```python
from build123d import *

# Parameters (mm, degrees)
SKETCH1_W           = 150
SKETCH1_H           = 150
SKETCH1_W_2         = 140
SKETCH1_H_2         = 140
BOSS_EXTRUDE1_DEPTH = 80
BOSS_EXTRUDE2_DEPTH = 2
CIRPATTERN1_COUNT   = 4
CUT_EXTRUDE1_DEPTH  = 10


with BuildPart() as part:
    # Sketch1 → Boss-Extrude1 (new body)
    with BuildSketch(Plane(origin=(0, 91.979453816, 0), x_dir=(1, 0, 0), z_dir=(0, 1, 0))):
        with Locations((62.661143414, -111.558685069)):
            Rectangle(SKETCH1_W, SKETCH1_H)
        with Locations((62.661143414, -111.558685069)):
            Rectangle(SKETCH1_W_2, SKETCH1_H_2, mode=Mode.SUBTRACT)
    extrude(amount=BOSS_EXTRUDE1_DEPTH)

    # Sketch5 → Boss-Extrude2 (add)
    with BuildSketch(Plane.XZ.offset(-91.979453816)):
        with BuildLine():
            Line((-8.863856586, 184.058685069), (-8.863856586, 39.058685069))
            ThreePointArc((-8.863856586, 39.058685069), (-9.838856586, 38.083685069), (-10.813856586, 39.058685069))
            Line((-10.813856586, 39.058685069), (-10.813856586, 184.058685069))
            ThreePointArc((-10.813856586, 184.058685069), (-9.838856586, 185.033685069), (-8.863856586, 184.058685069))
        make_face()
    boss_extrude2 = extrude(amount=BOSS_EXTRUDE2_DEPTH)

    # CirPattern1: Boss-Extrude2 ×4 about axis
    cirpattern1_axis = Axis((62.661143414, 0, 111.558685069), (0, 1, 0))
    for i in range(1, CIRPATTERN1_COUNT):
        add(boss_extrude2.rotate(cirpattern1_axis, i * 360 / CIRPATTERN1_COUNT))

    # Sketch6 → Cut-Extrude1 (cut)
    with BuildSketch(Plane(origin=(0, 0, 36.558685069), x_dir=(-1, 0, 0), z_dir=(0, 0, -1))):
        with BuildLine():
            Line((-67.328548343, 91.979453816), (-67.328548343, 106.844407314))
            ThreePointArc((-67.328548343, 106.844407314), (-62.661143414, 111.511812242), (-57.993738486, 106.844407314))
            Line((-57.993738486, 106.844407314), (-57.993738486, 91.979453816))
            Line((-57.993738486, 91.979453816), (-57.993738486, 79.02025395))
            Line((-57.993738486, 79.02025395), (-67.328548343, 79.02025395))
            Line((-67.328548343, 79.02025395), (-67.328548343, 91.979453816))
        make_face()
    extrude(amount=-CUT_EXTRUDE1_DEPTH, mode=Mode.SUBTRACT)


solid = part.part
```
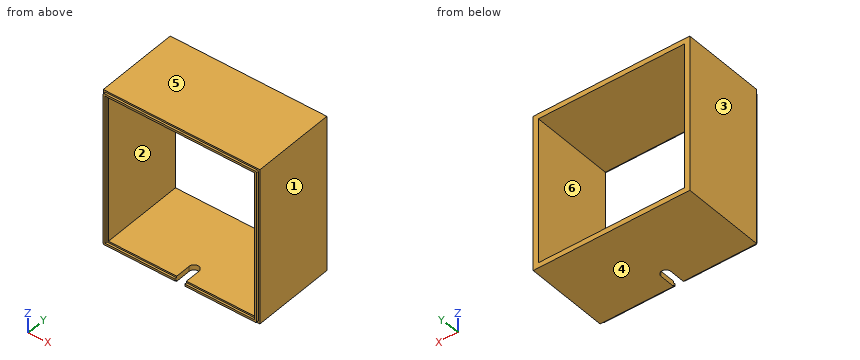
The model under review builds one solid part; all positions refer to its coordinate system, in mm. Face numbers are marked on the shaded views. A direction names the side the tool comes from. Round coordinates to 2 decimals unless told otherwise and drop trailing zeros. Write each loop counter-clockwise with the first axis right and the second up, starting at its lowest first coordinate (ties: lowest second). Pieces come first, ordered by that corner, then holes. Notation, with made-up numbers: M 15.25,-11.75 L 57.25,-11.75 A10 ccw 57.25,5.25 Z; hole C 25.25,57 d4. An arc over 180 degrees is marked long. Use CSV: the item, a comma, the result in double quotes. Start each with the question number.
(1) We need section C-C, the plane y = 144.5. State the section outline as (x, z) points, then the cut area to 3 significant figures.
(2) Clearance check with flat-ended pins moving along their axes: P1, Ø1, axis at x = 29.5, y = 90.5, coming from the -Z side; P2, Ø0.6, axis at y = 90.5, z = 75.5, coming from the +X side; P3, Ø0.6, axis at x = 91, y = 91, coming from the +Z side. State where each tip first meets the part, or that it passes through.
(3) We need section A-A, the plane x = 41. State the section outline as (y, z) points, then the cut area to 3 significant figures.
(4) For line 1 along Z through (x, y) = (37, 148); line 2 along X through (y, z) = (100.5, 110.5), list the stretches that pass through material, from the lowest coordinate up.
(5) We need section B-B, the plane z = 97.5. State the section outline as (x, y) points, then the cut area to 3 significant figures.
(6) Tool access review of the marked faces 5 and 6: name each direction out of +Z, -Z, +X, -X, +Y, -Y from which nothing blocks a thin tool from reaching the whole face with its end or side.
(7) The part is to be moulded in two halves that separate along X. For the marked faces 1, 2, 3 and 4, say which applies: +X half, -X half, draft (parallel to the pull), parting line (faces both ways), or undercut.
Findings:
1,outline,"M -12.34,36.56 L 137.66,36.56 L 137.66,186.56 L -12.34,186.56 Z; hole M -7.34,41.56 L 132.66,41.56 L 132.66,181.56 L -7.34,181.56 Z"
1,area,"2,900 mm^2"
2,P1,"z = 38.08"
2,P2,"x = 136.14"
2,P3,"z = 185.03"
3,outline,"M 89.98,38.08 L 91.98,38.08 L 91.98,36.56 L 171.98,36.56 L 171.98,41.56 L 91.98,41.56 L 91.98,40.03 L 89.98,40.03 Z; M 89.98,183.08 L 91.98,183.08 L 91.98,181.56 L 171.98,181.56 L 171.98,186.56 L 91.98,186.56 L 91.98,185.03 L 89.98,185.03 Z"
3,area,"808 mm^2"
4,line 1,"36.56 to 41.56, 181.56 to 186.56"
4,line 2,"-12.34 to -7.34, 132.66 to 137.66"
5,outline,"M -12.34,91.98 L -10.81,91.98 L -10.81,89.98 L -8.86,89.98 L -8.86,91.98 L -7.34,91.98 L -7.34,171.98 L -12.34,171.98 Z; M 132.66,91.98 L 134.19,91.98 L 134.19,89.98 L 136.14,89.98 L 136.14,91.98 L 137.66,91.98 L 137.66,171.98 L 132.66,171.98 Z"
5,area,"808 mm^2"
6,face 5,"+Z, +X, -X, +Y, -Y"
6,face 6,"+Y, -Y"
7,face 1,"+X half"
7,face 2,"undercut"
7,face 3,"-X half"
7,face 4,"draft"
